```python
from build123d import *

# Parameters (mm, degrees)
EXTRUDE_1_DEPTH     = 25
SKETCH_2_R          = 1.7
CUT_EXTRUDE_1_DEPTH = 25
SKETCH_3_R          = 2.75
CUT_EXTRUDE_2_DEPTH = 7.5
CUT_EXTRUDE_START   = -25
SKETCH_3_2_R        = 2.75
CUT_EXTRUDE_3_DEPTH = 7.5


with BuildPart() as part:
    # 草图1 → 凸台-拉伸1 (new body)
    with BuildSketch(Plane.XY):
        with BuildLine():
            Line((0, -2.75), (-15.2, -2.75))
            Line((-15.2, -2.75), (-15.2, -1.75))
            Line((-15.2, -1.75), (-2.121320344, -1.75))
            ThreePointArc((-2.121320344, -1.75), (1.17260394, 2.487468593), (0, -2.75))
        make_face()
    extrude(amount=EXTRUDE_1_DEPTH)

    # 草图2 → 切除-拉伸1 (cut)
    with BuildSketch(Plane(origin=(0, -1.75, 0), x_dir=(1, 0, 0), z_dir=(0, 1, 0))):
        with Locations((-10.4, -5.5)):
            Circle(SKETCH_2_R)
        with Locations((-10.4, -19.5)):
            Circle(SKETCH_2_R)
    extrude(amount=-CUT_EXTRUDE_1_DEPTH, mode=Mode.SUBTRACT)

    # 草图3 → 切除-拉伸2 (cut)
    with BuildSketch(Plane(origin=(0, 0, 0), x_dir=(-1, 0, 0), z_dir=(0, 0, -1))):
        Circle(SKETCH_3_R)
    extrude(amount=-CUT_EXTRUDE_2_DEPTH, mode=Mode.SUBTRACT)

    # 草图3<2> → 切除-拉伸3 (cut)
    with BuildSketch(Plane(origin=(0, 0, 0), x_dir=(-1, 0, 0), z_dir=(0, 0, -1)).offset(CUT_EXTRUDE_START)):
        Circle(SKETCH_3_2_R)
    extrude(amount=CUT_EXTRUDE_3_DEPTH, mode=Mode.SUBTRACT)


solid = part.part
```
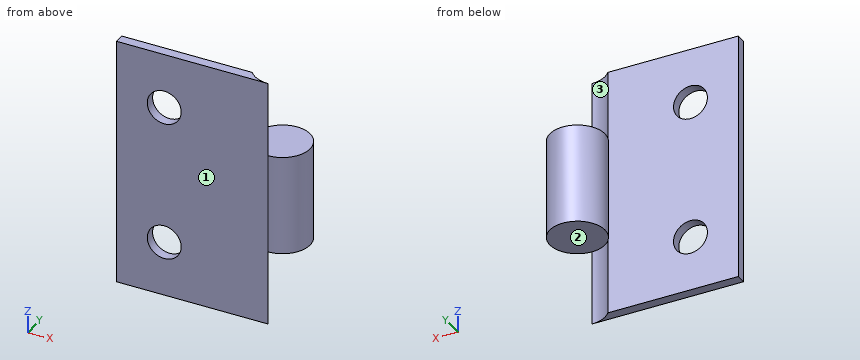
Read the model definition and answer for the solid it produces. Units are mm, in the model's axes. Face numbers are marked on the shaded views. A direction names the side the tool comes from. Round coordinates to 2 decimals unless told otherwise and drop trailing zeros. Write each loop counter-clockwise with the first axis right and the second up, starting at its lowest first coordinate (ties: lowest second). Pieces come first, ordered by that corner, then holes. Notation, with made-up numbers: M 66.25,13 L 72.25,13 A16 cw 72.25,28 Z; hole C 33.25,16.5 d9. An arc over 180 degrees is marked long. One line per item, written item: value.
Q1. Find section A-A on z = 5.5. Write down the section's boundary in (x, y), plus the area to 3 significant figures.
Data:
outline: M -15.2,-2.75 L -12.1,-2.75 L -12.1,-1.75 L -15.2,-1.75 Z; M -8.7,-2.75 L 0,-2.75 A2.75 cw -2.12,-1.75 L -8.7,-1.75 Z
area: 10.3 mm2
Q2. Find section C-C on y = -2.2. Write down the section's boundary in (x, z), plus the area to 3 significant figures.
Data:
outline: M -15.2,0 L -1.65,0 L -1.65,7.5 L 1.65,7.5 L 1.65,17.5 L -1.65,17.5 L -1.65,25 L -15.2,25 Z; hole C -10.4,5.5 d3.4; hole C -10.4,19.5 d3.4
area: 354 mm2
Q3. Find section B-B on x = -9.25. Write down the section's boundary in (y, z), plus the area to 3 significant figures.
Data:
outline: M -2.75,0 L -1.75,0 L -1.75,4.25 L -2.75,4.25 Z; M -2.75,6.75 L -1.75,6.75 L -1.75,18.25 L -2.75,18.25 Z; M -2.75,20.75 L -1.75,20.75 L -1.75,25 L -2.75,25 Z
area: 20.0 mm2
Q4. Which of the six approach directions +Z, -Z, +X, -X, +Y, -Y give full straight-line access (tool end or side, diameter ignored) to the marked faces 1, 2 and 3?
Data:
face 1: +Z, -Z, +X, -X, -Y
face 2: -Z, +X, +Y
face 3: +Z, +X, +Y
Q5. Flat-ended cylindrical pins translate along their axes: pin 1 Ø3 at (x, y) = (-1.5, 0.5) entering from +Z; pin 2 Ø1.5 at (x, y) = (0, 1) entering from -Z; pin 3 Ø5.5 at (x, z) = (-10.4, 5.5) entering from +Y. Find the tip coordinate at first contact, or state that the pin passes through.
Data:
pin 1: z = 17.5
pin 2: z = 7.5
pin 3: y = -1.75
Q6. Find section D-D on x = -1.75. Write down the section's boundary in (y, z).
Data:
outline: M -2.75,0 L -2.12,0 L -2.12,7.5 L 2.12,7.5 L 2.12,17.5 L -2.12,17.5 L -2.12,25 L -2.75,25 Z
Q7. Straight lines are drawn through the part: line 1 (Z direction, x = -10.4, y = -2.1); line 2 (Z direction, x = -1, y = -2); line 3 (Y direction, x = -12.25, z = 17). For each, find the intervals that lie inside material, in ascending order. Write a range as [from, to].
Data:
line 1: [0, 3.8], [7.2, 17.8], [21.2, 25]
line 2: [7.5, 17.5]
line 3: [-2.75, -1.75]
